```python
from build123d import *

# Parameters (mm, degrees)
F0_W     = 92
F0_H     = 50
F0_R     = 2.25
F0_R_2   = 1.75
F0_W_2   = 40
F1_DEPTH = 2
F2_R     = 3
F3_R     = 1.5


# Not quite as in the source:
# - a feature names something its author has since deleted; it is built from what else it names


with BuildPart() as f1:
    # F0 (on Front) → F1 (new body)
    with BuildSketch(Plane.XZ):
        with Locations((46, 25)):
            Rectangle(F0_W, F0_H)
        with Locations((5, 5)):
            Circle(F0_R, mode=Mode.SUBTRACT)
        with Locations((87, 5)):
            Circle(F0_R, mode=Mode.SUBTRACT)
        with BuildLine():
            Line((8.5, 27), (14, 27))
            Line((14, 27), (14, 32.5))
            ThreePointArc((14, 32.5), (16, 34.5), (18, 32.5))
            Line((18, 32.5), (18, 27))
            Line((18, 27), (23.5, 27))
            ThreePointArc((23.5, 27), (25.5, 25), (23.5, 23))
            Line((23.5, 23), (18, 23))
            Line((18, 23), (18, 17.5))
            ThreePointArc((18, 17.5), (16, 15.5), (14, 17.5))
            Line((14, 17.5), (14, 23))
            Line((14, 23), (8.5, 23))
            ThreePointArc((8.5, 23), (6.5, 25), (8.5, 27))
        make_face(mode=Mode.SUBTRACT)
        with Locations((46, 25)):
            Circle(F0_R_2, mode=Mode.SUBTRACT)
        with Locations((5, 45)):
            Circle(F0_R, mode=Mode.SUBTRACT)
        with Locations((87, 45)):
            Circle(F0_R, mode=Mode.SUBTRACT)
        with Locations((112, 25)):
            Rectangle(F0_W_2, F0_H)
        with BuildLine():
            Line((114, 27), (114, 32.5))
            ThreePointArc((114, 32.5), (116, 34.5), (118, 32.5))
            Line((118, 32.5), (118, 27))
            Line((118, 27), (123.5, 27))
            ThreePointArc((123.5, 27), (125.5, 25), (123.5, 23))
            Line((123.5, 23), (118, 23))
            Line((118, 23), (118, 17.5))
            ThreePointArc((118, 17.5), (116, 15.5), (114, 17.5))
            Line((114, 17.5), (114, 23))
            Line((114, 23), (108.5, 23))
            ThreePointArc((108.5, 23), (106.5, 25), (108.5, 27))
            Line((108.5, 27), (114, 27))
        make_face(mode=Mode.SUBTRACT)
    extrude(amount=F1_DEPTH)

    # F2
    f2_edges = [f1.edges().sort_by_distance(p)[0] for p in [
        (14, -1, 27),
        (14, -1, 23),
        (18, -1, 27),
        (18, -1, 23),
        (114, -1, 27),
        (118, -1, 27),
        (114, -1, 23),
        (118, -1, 23),
    ]]
    fillet(f2_edges, radius=F2_R)

    # F3
    f3_edges = [f1.edges().sort_by_distance(p)[0] for p in [
        (0, -1, 50),
        (0, -1, 0),
        (132, -1, 0),
        (132, -1, 50),
    ]]
    fillet(f3_edges, radius=F3_R)


solid = f1.part
```
For this review, take the finished solid that the model builds, in its own axes (mm). A direction names the side the tool comes from. Coordinates: 2 decimals unless noted, no trailing zeros. Order: outer loops, then holes, each group sorted by start corner. A loop starts at its lowest first (then second) coordinate and runs counter-clockwise, first axis right, second up. Notation, with made-up numbers: (13.5, 1) -> (27.5, 1) arc R29 cw to (27.5, 36) -> close; hole circle Ø7 at (-1, 21.25). An arc over 180 degrees is marked (long way). Answer as CSV lines item,"result".
Q1. We need section C-C (z = 25). State the section outline as (x, y) points.
Model answer:
outline,"(0, -2) -> (6.5, -2) -> (6.5, 0) -> (0, 0) -> close; (25.5, -2) -> (44.25, -2) -> (44.25, 0) -> (25.5, 0) -> close; (47.75, -2) -> (106.5, -2) -> (106.5, 0) -> (47.75, 0) -> close; (125.5, -2) -> (132, -2) -> (132, 0) -> (125.5, 0) -> close"
Q2. For faces 1 (the face through (118.86, -1.01, 22.1)), 2 (the face through (65, -2, 25)), list the 3-axis set-ups (+Z, -Z, +X, -X, +Y, -Y) from which the entire face can be reached by the end or side of a thin tool; tool diameter is ignored.
Model answer:
face 1,"+Y, -Y"
face 2,"+Z, -Z, +X, -X, -Y"
Q3. We need section D-D (y = -1.65). Count the separate pieces of the cut face and the enclosed holes in it, plus the area to 3 significant figures.
Model answer:
separate pieces,"1"
enclosed holes,"7"
area,"6,250 mm2"
Q4. We need section A-A (x = 87). State the section outline as (y, z) points, plus the area to 3 significant figures.
Model answer:
outline,"(-2, 0) -> (0, 0) -> (0, 2.75) -> (-2, 2.75) -> close; (-2, 7.25) -> (0, 7.25) -> (0, 42.75) -> (-2, 42.75) -> close; (-2, 47.25) -> (0, 47.25) -> (0, 50) -> (-2, 50) -> close"
area,"82.0 mm2"
Q5. Wall thickness on line 1 along Z through (x, y) = (5, -0.4); line 2 along Z through (x, y) = (46, -0.7); line 3 along X through (y, z) = (-0.05, 16): over which ranges is each line inside the solid? List them lowest first. Write a range as [from, to].
Model answer:
line 1,"z = [0, 2.75], [7.25, 42.75], [47.25, 50]"
line 2,"z = [0, 23.25], [26.75, 50]"
line 3,"x = [0, 14.68], [17.32, 114.68], [117.32, 132]"
Q6. We need section B-B (x = 16). State the section outline as (y, z) points.
Model answer:
outline,"(-2, 0) -> (0, 0) -> (0, 15.5) -> (-2, 15.5) -> close; (-2, 34.5) -> (0, 34.5) -> (0, 50) -> (-2, 50) -> close"
Q7. Draft analysis for pull direction X (two halves, no side actions). For faces 3 (the face through (4.71, -0.99, 47.23)), 4 (the face through (65, 0, 25)), 5 (the face through (89.08, -0.99, 4.14)), state which applies: released by +X, released by -X, zero draft, split by the parting line, or undercut.
Model answer:
face 3,"undercut"
face 4,"zero draft"
face 5,"undercut"
